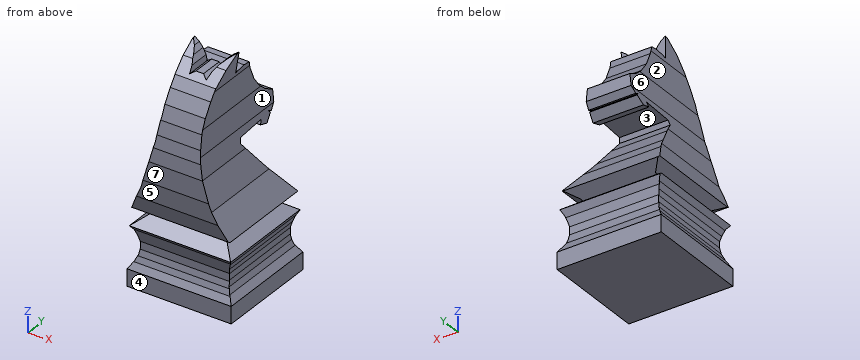
```python
from build123d import *

# Parameters (mm, degrees)
F2_W     = 43.18
F2_H     = 86.36
F3_DEPTH = 21.59
F4_W     = 43.18
F4_H     = 86.36
F5_DEPTH = 43.18
F7_DEPTH = 21.59


with BuildPart() as f3:
    # F2 (on Right) → F3 (new body, symmetric)
    with BuildSketch(Plane.YZ):
        Rectangle(F2_W, F2_H)
    extrude(amount=F3_DEPTH, both=True)

    # F4 (on face) → F5 (cut)
    with BuildSketch(Plane(origin=(0, 21.59, 0), x_dir=(-1, 0, 0), z_dir=(0, 1, 0))):
        Rectangle(F4_W, F4_H)
        Polygon((18.302919, -40.662199), (-18.461943, -40.662199), (-18.438558, -34.686282), (-16.829565, -32.120593), (-16.069479, -30.044995), (-15.809655, -28.096024), (-15.809655, -25.911188), (-16.199389, -24.026766), (-16.846587, -22.005791), (-17.888235, -20.094059), (-13.049044, -16.243285), (-17.206199, -13.921896), (-12.399486, -4.064204), (-9.379052, 5.809045), (-7.917551, 12.629382), (-7.105607, 20.618919), (-7.105607, 30.557126), (-7.950029, 38.806483), (-6.30046, 37.604805), (-4.702249, 36.110826), (-3.533049, 34.194637), (-3.045882, 32.37588), (-1.292081, 33.382691), (1.371098, 33.382691), (2.897554, 32.37588), (3.384721, 34.194637), (4.5864, 36.110826), (5.982945, 37.604805), (7.736745, 38.806483), (7.184624, 30.557126), (7.184624, 20.618919), (7.964091, 12.629382), (9.523025, 5.809045), (12.510981, -4.064204), (17.273372, -13.921896), (13.01294, -16.243285), (17.901512, -20.094059), (16.727163, -22.005791), (15.989779, -24.026766), (15.607432, -25.911188), (15.607432, -28.096024), (15.889227, -30.044995), (16.763162, -32.120593), (18.302919, -34.686282), align=None, mode=Mode.SUBTRACT)
    extrude(amount=-F5_DEPTH, mode=Mode.SUBTRACT)

    # F6 (on Right) → F7 (cut, symmetric)
    with BuildSketch(Plane.YZ):
        Polygon((18.948087, -40.815897), (22.037912, -40.815897), (22.175604, 40.474616), (-21.876609, 40.474616), (-21.876609, -40.680926), (-17.684452, -40.680926), (-17.684452, -34.686282), (-16.250653, -32.487791), (-15.455558, -30.56524), (-14.857819, -28.473156), (-14.857819, -25.76942), (-16.058451, -21.550797), (-17.192863, -20.088844), (-12.195049, -16.210757), (-17.110933, -13.534333), (-18.558385, -8.031274), (-19.268457, -1.271935), (-19.268457, 5.774164), (-18.653972, 10.635425), (-17.757623, 14.789965), (-16.455481, 19.347463), (-14.502783, 23.826377), (-11.717116, 28.127776), (-9.24552, 31.391378), (-4.643708, 35.474289), (0.57259, 38.628653), (1.528456, 38.765203), (0.873005, 31.732757), (1.719629, 31.964898), (5.078816, 32.38821), (7.72793, 32.101449), (8.465313, 29.43868), (10.418011, 24.932453), (13.094435, 21.300161), (15.962034, 18.719323), (19.389497, 16.971454), (19.389497, 12.779298), (17.573351, 10.853911), (16.073769, 11.526532), (16.980739, 10.580613), (14.528235, 8.229095), (11.469464, 9.103029), (12.275122, 10.550483), (1.446525, 9.813101), (0.833981, 8.242985), (3.885183, 4.380703), (8.519922, -1.683081), (12.478762, -6.626802), (18.445989, -14.177564), (13.676071, -16.514244), (18.697038, -20.395836), (17.248681, -22.751831), (16.360357, -25.687164), (16.360357, -28.410073), (17.036257, -31.364718), (18.948087, -34.686282), align=None)
    extrude(amount=F7_DEPTH, both=True, mode=Mode.SUBTRACT)


solid = f3.part
```
Input: part model. Units: mm. Frame: model coordinates. Face numbers are marked on the shaded views. A direction names the side the tool comes from. Round coordinates to 2 decimals unless told otherwise and drop trailing zeros. Loops run counter-clockwise (first coordinate to the right, second up) from the corner with the lowest first, then second, coordinate; pieces in that order, holes last.
1) Set-up query: the marked faces 1, 2, 3 and 4. Return all of +Z, -Z, +X, -X, +Y, -Y with unobstructed straight access to the full face (end or side cutting, diameter ignored); none if empty.
Ans:
face 1: +X, +Y, -Y
face 2: -X, +Y, -Y
face 3: +X, -X
face 4: -Z, +X, -X, -Y
2) Pin query (flat end, axial travel): pin 1 (2.5 mm diameter, centred on y = 3.5, z = -27.5, fed in from -X); pin 2 (1.5 mm diameter, centred on x = -7.5, y = -4, fed in from +Z); pin 3 (8 mm diameter, centred on y = 1, z = 27.5, fed in from -X). Return the tip coordinate at first contact, or that it passes through.
Ans:
pin 1: stops at x = -15.7
pin 2: stops at z = 36.32
pin 3: stops at x = -7.25
3) Pull-direction query (Z, two-part tool) for the marked faces 5, 6 and 7; classes: released by +Z, released by -Z, zero draft, split by the parting line, or undercut.
Ans:
face 5: released by -Z
face 6: undercut
face 7: zero draft
4) Section query B-B on z = 3.5. Return the cut outline in (x, y), plus the area to 3 significant figures.
Ans:
outline: (-10.22, -19.27) - (10.09, -19.27) - (10.09, 4.56) - (-10.22, 4.56) - close
area: 484 mm2
5) Material intervals for line 1 (Z direction, x = 16, y = 18); line 2 (Y direction, x = -15, z = -30.5); line 3 (X direction, y = -0.5, z = 20.5), sorted ascending.
Ans:
line 1: z = -40.66 to -33.04, -21.53 to -19.86, -14.4 to -13.61
line 2: y = -15.44 to 16.84
line 3: x = -7.2 to 7.12
